Work out the finished part from the listing and answer in its coordinate system (mm). Coordinates: 2 decimals unless noted, no trailing zeros. Loops run counter-clockwise (first coordinate to the right, second up) from the corner with the lowest first, then second, coordinate; pieces in that order, holes last. Notation, with made-up numbers: (62.5, -29) -> (112.5, -29) arc R36 cw to (112.5, 5) -> close; hole circle Ø5 at (-36, -10.5). An arc over 180 degrees is marked (long way). Answer as CSV lines item,"result".
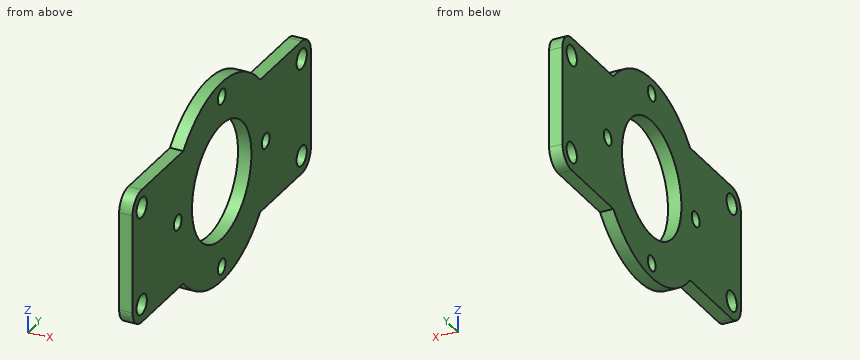
```python
from build123d import *

# Parameters (mm, degrees)
SKETCH_1_W          = 3
SKETCH_1_H          = 30
EXTRUDE_1_DEPTH     = 78
SKETCH_2_R          = 22.5
EXTRUDE_2_DEPTH     = 3
SKETCH_3_R          = 13
CUT_EXTRUDE_1_DEPTH = 87.598210143
HOLE_WIZARD_M31_D   = 3.4
HOLE_WIZARD_M41_D   = 4.5
FILLET_1_R          = 4


with BuildPart() as part:
    # Эскиз1 → Бобышка-Вытянуть1 (new body)
    with BuildSketch(Plane(origin=(0, 0, 0), x_dir=(1, 0, 0), z_dir=(0, 1, 0))):
        with Locations((1.5, -15)):
            Rectangle(SKETCH_1_W, SKETCH_1_H)
    extrude(amount=EXTRUDE_1_DEPTH)

    # Эскиз2 → Бобышка-Вытянуть2 (add)
    with BuildSketch(Plane.ZY):
        with Locations((15, 39)):
            Circle(SKETCH_2_R)
    extrude(amount=-EXTRUDE_2_DEPTH)

    # Эскиз3 → Вырез-Вытянуть1 (cut, through all)
    with BuildSketch(Plane.ZY):
        with Locations((15, 39)):
            Circle(SKETCH_3_R)
    extrude(amount=-CUT_EXTRUDE_1_DEPTH, mode=Mode.SUBTRACT)

    # Отверстие с зазором M31 (through all)
    with Locations(Plane(origin=(3, -25.024735225, 7.262908886), x_dir=(0, 0, 1), z_dir=(1, 0, 0))):
        with Locations((7.737091114, -83.274735225), (-11.512908886, -64.024735225), (7.737091114, -44.774735225), (26.987091114, -64.024735225)):
            Hole(HOLE_WIZARD_M31_D / 2)

    # Отверстие с зазором M41 (through all)
    with Locations(Plane(origin=(3, 0, 0), x_dir=(0, 0, -1), z_dir=(1, 0, 0))):
        with Locations((-26, 74), (-4, 74), (-4, 4), (-26, 4)):
            Hole(HOLE_WIZARD_M41_D / 2)

    # Скругление1
    fillet_1_edges = [part.edges().sort_by_distance(p)[0] for p in [
        (1.5, 78, 0),
        (1.5, 0, 0),
        (1.5, 0, 30),
        (1.5, 78, 30),
    ]]
    fillet(fillet_1_edges, radius=FILLET_1_R)


solid = part.part
```
(1) A cutting plane is placed at C-C, the plane x = 2. Count the separate pieces of the cut face and the enclosed holes in it, and give its area (3 significant figures).
Computed values:
separate pieces,"1"
enclosed holes,"9"
area,"2,040 mm2"
(2) A cutting plane is placed at A-A, the plane z = 15. Write down the section's boundary in (x, y), and give its area (3 significant figures).
Computed values:
outline,"(0, 0) -> (3, 0) -> (3, 18.05) -> (0, 18.05) -> close; (0, 21.45) -> (3, 21.45) -> (3, 26) -> (0, 26) -> close; (0, 52) -> (3, 52) -> (3, 56.55) -> (0, 56.55) -> close; (0, 59.95) -> (3, 59.95) -> (3, 78) -> (0, 78) -> close"
area,"136 mm2"
(3) A flat-ended cylindrical pin translates along its axis: pin 1 Ø1.5 at (x, y) = (2, 9.5) entering from -Z. Find the tip coordinate at first contact, or state that the pin passes through.
Computed values:
pin 1,"z = 0"
(4) Consider line 1 along Y through (x, z) = (0.8, 15); line 2 along Z through (x, y) = (1.3, 72); line 3 along Y through (x, z) = (2.15, 4). Determine where each line is inside the solid, lowest interval first.
Computed values:
line 1,"0 to 18.05, 21.45 to 26, 52 to 56.55, 59.95 to 78"
line 2,"0 to 2.97, 5.03 to 24.97, 27.03 to 30"
line 3,"0 to 1.75, 6.25 to 32.07, 45.93 to 71.75, 76.25 to 78"
(5) A cutting plane is placed at D-D, the plane z = -4.25. Write down the section's boundary in (x, y), and give its area (3 significant figures).
Computed values:
outline,"(0, 27.35) -> (3, 27.35) -> (3, 37.3) -> (0, 37.3) -> close; (0, 40.7) -> (3, 40.7) -> (3, 50.65) -> (0, 50.65) -> close"
area,"59.7 mm2"
(6) A cutting plane is placed at B-B, the plane y = 19.75. Write down the section's boundary in (x, z).
Computed values:
outline,"(0, 0) -> (3, 0) -> (3, 13.3) -> (0, 13.3) -> close; (0, 16.7) -> (3, 16.7) -> (3, 30) -> (0, 30) -> close"
